from build123d import *

# Parameters (mm, degrees)
F0_W     = 100
F0_H     = 100
F1_DEPTH = 100
F2_R     = 5
F3_DEPTH = 10
F4_R     = 5
F5_DEPTH = 107.80932
F6_R     = 5
F7_DEPTH = 333.937347


with BuildPart() as f1:
    # F0 (on Front) → F1 (new body)
    with BuildSketch(Plane.XZ):
        with Locations((50, 50)):
            Rectangle(F0_W, F0_H)
    extrude(amount=F1_DEPTH)

    # F2 (on Top) → F3 (join)
    with BuildSketch(Plane.XY):
        with Locations((48.760578, -47.517374)):
            Circle(F2_R)
    extrude(amount=-F3_DEPTH)

    # F4 (on Top) → F5 (join)
    with BuildSketch(Plane.XY):
        with Locations((38.912062, -49.283471)):
            Circle(F4_R)
    extrude(amount=F5_DEPTH)

    # F6 (on Right) → F7 (cut)
    with BuildSketch(Plane.YZ):
        with Locations((-49.518168, 49.6369)):
            Circle(F6_R)
    extrude(amount=F7_DEPTH, mode=Mode.SUBTRACT)


solid = f1.part
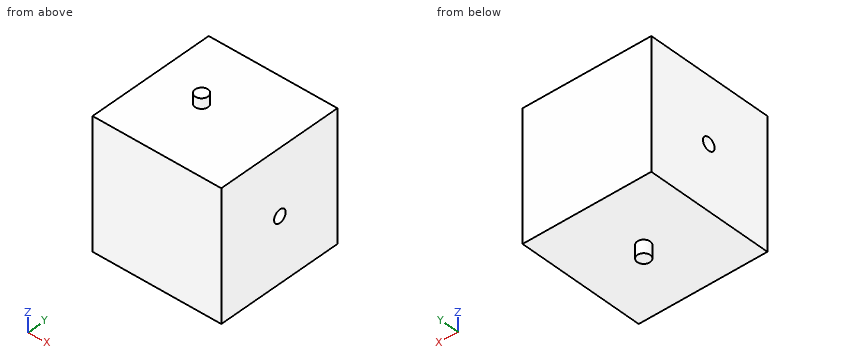
Design review of the part built by this model. Coordinates are the model's own, in mm. Give positions to 0.01 mm unless a question says otherwise; leave off trailing zeros. Write each loop counter-clockwise with the first axis right and the second up, starting at its lowest first coordinate (ties: lowest second). Pieces come first, ordered by that corner, then holes. Notation, with made-up numbers: M 72,81.5 L 130,81.5 A8 ccw 130,94.5 Z; hole C -31,77 d8. An arc over 180 degrees is marked long. Answer as a JSON object with one key per item and string values. Group by question number.
1) We need section B-B (x = 48). Give the boundary of the cut face in (y, z).
2) We need section A-A (z = 51.5). Give the boundary of the cut face in (x, y).
3) We need section C-C (y = -79). Give the boundary of the cut face in (x, z).
4) For line 1 along Z through (x, y) = (45, -21); line 2 along Y through (x, z) = (34.5, 53); line 3 along Z through (x, y) = (72, -45.5), list the stretches that pass through material, from the lowest coordinate up.
5) We need section D-D (x = 64.5). Give the boundary of the cut face in (y, z), and give its area (3 significant figures).
Answer key:
{
 "1": {"outline": "M -100,0 L -52.46,0 L -52.46,-10 L -42.58,-10 L -42.58,0 L 0,0 L 0,100 L -100,100 Z; hole C -49.52,49.64 d10"},
 "2": {"outline": "M 0,-100 L 100,-100 L 100,-54.16 L 0,-54.16 Z; M 0,-44.88 L 100,-44.88 L 100,0 L 0,0 Z"},
 "3": {"outline": "M 0,0 L 100,0 L 100,100 L 0,100 Z"},
 "4": {"line 1": "z = 0 to 100", "line 2": "y = -100 to -53.22, -45.82 to 0", "line 3": "z = 0 to 46.66, 52.61 to 100"},
 "5": {"outline": "M -100,0 L 0,0 L 0,100 L -100,100 Z; hole C -49.52,49.64 d10", "area": "9,920 mm²"}
}
